```python
from build123d import *

# Parameters (mm, degrees)
ESQUISSE1_R             = 5.5
ESQUISSE1_R_2           = 2.5
BOSS_EXTRU_1_DEPTH      = 20
ENL_V_MAT_EXTRU_1_DEPTH = 10


with BuildPart() as part:
    # Esquisse1 → Boss.-Extru.1 (new body)
    with BuildSketch(Plane(origin=(0, 0, 0), x_dir=(1, 0, 0), z_dir=(0, 1, 0))):
        with Locations(Location((0, 0, 0), (0, 0, 270))):
            Circle(ESQUISSE1_R)
        with Locations(Location((0, 0, 0), (0, 0, 270))):
            Circle(ESQUISSE1_R_2, mode=Mode.SUBTRACT)
    extrude(amount=BOSS_EXTRU_1_DEPTH)

    # Esquisse2 → Enlèv. mat.-Extru.1 (cut)
    with BuildSketch(Plane(origin=(0, 20, 0), x_dir=(1, 0, 0), z_dir=(0, 1, 0))):
        Polygon((-1.5, 5.80668977), (-1.5, 1.5), (-8.808638821, 1.5), (-9.18844746, -1.5), (-1.5, -1.5), (-1.5, -5.792081745), (1.5, -5.792081745), (1.5, -1.5), (7.78364435, -1.5), (7.981313964, 1.5), (1.5, 1.5), (1.5, 5.80668977), align=None)
    extrude(amount=-ENL_V_MAT_EXTRU_1_DEPTH, mode=Mode.SUBTRACT)


solid = part.part
```
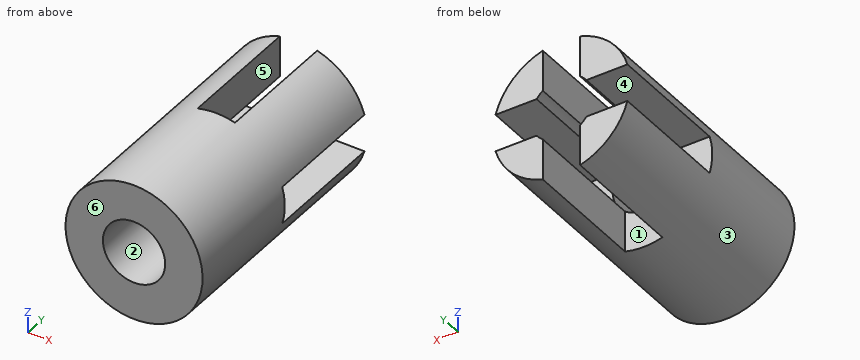
Geometry check sheet. Reference: the model listing, model coordinates, mm. Face numbers are marked on the shaded views. A direction names the side the tool comes from. Round coordinates to 2 decimals unless told otherwise and drop trailing zeros. Order: outer loops, then holes, each group sorted by start corner. A loop starts at its lowest first (then second) coordinate and runs counter-clockwise, first axis right, second up. Notation, with made-up numbers: (48.25, -14) - (98.25, -14) arc R19 ccw to (98.25, 13) - close; hole circle Ø5 at (-15.75, 26). An arc over 180 degrees is marked (long way). Use a Markdown table: item, result. Add a question column.
(1) Material ranges on line 1 along Z through (x, y) = (1.5, 5.75); line 2 along Z through (x, y) = (0, 5.75), recorded low to high. Write a range as [from, to].
(2) Sectioned sample at D-D, the plane y = 7.75. Enter the section's corners in (x, z), and give its area (3 significant figures).
(3) Depth check by flat-ended pin: pin 1 (6 mm diameter, centred on y = 17.5, z = -3, fed in from +X); pin 2 (1.6 mm diameter, centred on y = 17.5, z = 4, fed in from +X); pin 3 (1.5 mm diameter, centred on x = -0.5, z = 3, fed in from +Y). Enter the tip coordinate at first touch or a pass-through.
(4) Sectioned sample at C-C, the plane z = 0. Enter the section's corners in (x, y), and give its area (3 significant figures).
(5) Tool access check on the marked faces 4, 5 and 6. Record the directions out of +Z, -Z, +X, -X, +Y, -Y that give a thin tool (end or side, any length) a straight path to the whole face; none if there is none.
(6) Sectioned sample at A-A, the plane y = 10.5. Enter the section's corners in (x, z), and give its area (3 significant figures).
(7) Sectioned sample at B-B, the plane x = 0.25. Enter the section's corners in (y, z).
(8) Release check for a two-part mould opening along Z. For the marked faces 1, 2 and 3 record: pulls with the +Z half, pulls with the -Z half, needs draft (parallel to the pull), parting line crosses it, or undercut.
Answers below:
| question | item | result |
|---|---|---|
| 1 | line 1 | [-5.29, -2], [2, 5.29] |
| 1 | line 2 | [-5.5, -2.5], [2.5, 5.5] |
| 2 | outline | circle Ø11 at (0, 0); hole circle Ø5 at (0, 0) |
| 2 | area | 75.4 mm² |
| 3 | pin 1 | x = 5.29 |
| 3 | pin 2 | x = 4.47 |
| 3 | pin 3 | y = 10 |
| 4 | outline | (-5.5, 0) - (-2.5, 0) - (-2.5, 10) - (-5.5, 10) - close; (2.5, 0) - (5.5, 0) - (5.5, 10) - (2.5, 10) - close |
| 4 | area | 60.0 mm² |
| 5 | face 4 | +X, -X, +Y |
| 5 | face 5 | +Z, -Z, +Y |
| 5 | face 6 | +Z, -Z, +X, -X, -Y |
| 6 | outline | (-5.29, -1.5) arc R5.5 ccw to (-1.5, -5.29) - (-1.5, -2) arc R2.5 cw to (-2, -1.5) - close; (-5.29, 1.5) - (-2, 1.5) arc R2.5 cw to (-1.5, 2) - (-1.5, 5.29) arc R5.5 ccw to start; (1.5, -5.29) arc R5.5 ccw to (5.29, -1.5) - (2, -1.5) arc R2.5 cw to (1.5, -2) - close; (1.5, 2) arc R2.5 cw to (2, 1.5) - (5.29, 1.5) arc R5.5 ccw to (1.5, 5.29) - close |
| 6 | area | 38.3 mm² |
| 7 | outline | (0, -5.49) - (10, -5.49) - (10, -2.49) - (0, -2.49) - close; (0, 2.49) - (10, 2.49) - (10, 5.49) - (0, 5.49) - close |
| 8 | face 1 | needs draft |
| 8 | face 2 | undercut |
| 8 | face 3 | parting line crosses it |
